Input: dimensioned drawing with shaded views. Units: mm. Origin: part minimum x, y, z. Coordinates: 2 decimals unless noted, no trailing zeros. Write each loop counter-clockwise with the first axis right and the second up, starting at its lowest first coordinate (ties: lowest second). Pieces come first, ordered by that corner, then holes. Notation, with made-up numbers: (60, 41.25) -> (100, 41.25) arc R18 ccw to (100, 67.25) -> close; hole circle Ø1 at (49, 42.5). An arc over 180 degrees is marked (long way). One line per item, written item: value. Start each with the question number.
1. Section query A-A, the plane y = 13. Output: boundary loops of the cut face in (x, z), and give its area (4 significant figures).
2. Section query B-B, the plane z = 3.75. State how many separate pieces and enclosed holes the cut face has, and give its area (3 significant figures).
3. Section query D-D, the plane y = 25. Output: boundary loops of the cut face in (x, z).
4. Mould query, pull axis Y, two halves, no side actions, for the marked faces 1 and 2. Classes: released by +Y, released by -Y, zero draft, split by the parting line, or undercut.
5. Section query C-C, the plane x = 16. Output: boundary loops of the cut face in (y, z), and give its area (3 significant figures).
6. First-contact query: P1, Ø5, axis at x = 40, y = 48.5, coming from the +Z side; P2, Ø1, axis at y = 68, z = 5.5, coming from the -X side; P3, Ø2.5, axis at y = 57.5, z = 4, coming from the +X side. Flat tips, straight axial feed; report the tip coordinate or a pass-through.
7. Line query: line 1 (X direction, y = 65.5, z = 3); line 2 (X direction, y = 9, z = 4.25); line 3 (Y direction, x = 65, z = 3). Output: solid intervals per line, ascending.
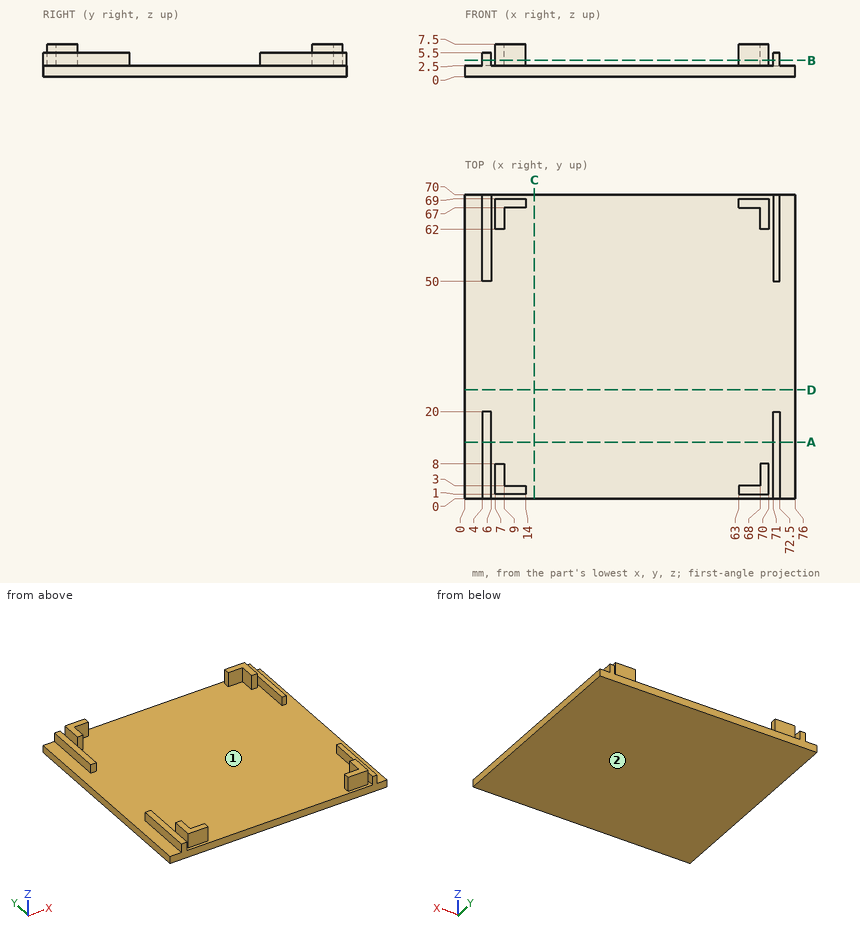
Computed values:
1. outline: (0, 0) -> (76, 0) -> (76, 2.5) -> (72.5, 2.5) -> (72.5, 5.5) -> (71, 5.5) -> (71, 2.5) -> (6, 2.5) -> (6, 5.5) -> (4, 5.5) -> (4, 2.5) -> (0, 2.5) -> close
1. area: 200.5 mm²
2. separate pieces: 8
2. enclosed holes: 0
2. area: 236 mm²
3. outline: (0, 0) -> (76, 0) -> (76, 2.5) -> (0, 2.5) -> close
4. face 1: undercut
4. face 2: zero draft
5. outline: (0, 0) -> (70, 0) -> (70, 2.5) -> (0, 2.5) -> close
5. area: 175 mm²
6. P1: stops at z = 2.5
6. P2: stops at x = 4
6. P3: stops at x = 72.5
7. line 1: x = 4 to 6, 7 to 9, 68 to 70, 71 to 72.5
7. line 2: x = 4 to 6, 71 to 72.5
7. line 3: y = 1 to 3, 67 to 69
